Autodesk Inventor part; units mm, degrees
ref_plane "YZ Plane" through (0, 0, 0) normal (1, 0, 0) x (0, 1, 0)
ref_plane "XZ Plane" through (0, 0, 0) normal (0, 1, 0) x (-1, 0, 0)
ref_plane "XY Plane" through (0, 0, 0) normal (0, 0, 1) x (1, 0, 0)
sketch "草圖8" plane through (0, 0, 0) normal (0, 1, 0) x (-1, 0, 0)
  line L0 (10, 10) -> (-10, 10)
  line L1 (-10, 10) -> (-10, -10)
  line L2 (-10, -10) -> (10, -10)
  line L3 (10, -10) -> (10, 10)
  line L4 (10, 10) -> (-10, -10) construction
  line L5 (-10, 10) -> (10, -10) construction
  point P0 (0, 0)
  dimension "d36" = 20
  dimension "d37" = 20
extrude "擠出8" add sketch "草圖8" along normal blind 1.5
sketch "草圖9" plane through (0, 1.5, 0) normal (0, 1, 0) x (1, 0, 0)
  line L0 (-8, -7) -> (8, -7)
  line L1 (8, -7) -> (8, 7)
  line L2 (8, 7) -> (-8, 7)
  line L3 (-8, 7) -> (-8, -7)
  line L4 (-8, -7) -> (8, 7) construction
  line L5 (8, -7) -> (-8, 7) construction
  line L6 (-7, 6) -> (7, 6)
  line L7 (7, 6) -> (7, -6)
  line L8 (7, -6) -> (-7, -6)
  line L9 (-7, -6) -> (-7, 6)
  line L10 (-7, 6) -> (7, -6) construction
  line L11 (7, 6) -> (-7, -6) construction
  point P0 (0, 0)
  dimension "d40" = 16
  dimension "d41" = 14
  dimension "d46" = 14
  dimension "d47" = 12
extrude "擠出10" add sketch "草圖9" along normal blind 15
sketch "草圖11" plane through (-8, 1.5, 7) normal (0, 0, 1) x (1, 0, 0)
  line L0 (5.5, 18) -> (10.5, 18)
  line L1 (10.5, 18) -> (10.5, 12)
  line L2 (10.5, 12) -> (5.5, 12)
  line L3 (5.5, 12) -> (5.5, 18)
  line L4 (16, 15) -> (0, 15)
  line L5 (5.5, 18) -> (10.5, 12) construction
  line L6 (10.5, 18) -> (5.5, 12) construction
  point P0 (8, -1.5)
  point P1 (8, 15)
  point P2 (10.5, 15)
  point P3 (5.5, 15)
  dimension "d50" = 5
  dimension "d51" = 6
extrude "擠出11" cut sketch "草圖11" against normal blind 15 contours L4 L1 L2 L3
sketch "草圖12" plane through (0, 1.5, 0) normal (0, 1, 0) x (1, 0, 0)
  line L0 (-4.5, 2.5) -> (-2.5, 2.5)
  line L1 (-2.5, 2.5) -> (-2.5, -2.5)
  line L2 (-2.5, -2.5) -> (-4.5, -2.5)
  line L3 (-4.5, -2.5) -> (-4.5, 2.5)
  line L4 (-4.5, 2.5) -> (-2.5, -2.5) construction
  line L5 (-2.5, 2.5) -> (-4.5, -2.5) construction
  line L6 (2.5, 2.5) -> (4.5, 2.5)
  line L7 (4.5, 2.5) -> (4.5, -2.5)
  line L8 (4.5, -2.5) -> (2.5, -2.5)
  line L9 (2.5, -2.5) -> (2.5, 2.5)
  line L10 (2.5, 2.5) -> (4.5, -2.5) construction
  line L11 (4.5, 2.5) -> (2.5, -2.5) construction
  line L12 (7, 6) -> (7, -6)
  point P0 (0, 0)
  point P1 (-3.5, 0)
  point P2 (3.5, 0)
  point P3 (7, 0)
  dimension "d54" = 5
  dimension "d55" = 2
  dimension "d56" = 5
  dimension "d57" = 2
  dimension "d58" = 3.5
  dimension "d59" = 3.5
  dimension "d60" = 3.5
extrude "擠出12" add sketch "草圖12" along normal blind 1
properties part number "差分線圈激勵"
Design review of the part built by this model. Coordinates are the model's own, in mm. A direction names the side the tool comes from. Give positions to 0.01 mm unless a question says otherwise; leave off trailing zeros. Write each loop counter-clockwise with the first axis right and the second up, starting at its lowest first coordinate (ties: lowest second). Pieces come first, ordered by that corner, then holes. Notation, with made-up numbers: M -8.75,-10.75 L 47.25,-10.75 A19 cw 47.25,2.25 Z; hole C -22,-19 d3. An arc over 180 degrees is marked long. Return JSON: item names as keys, results as strings. Group by question number.
Item 1: Take a section at B-B (y = 14.5). Give the boundary of the cut face in (x, z).
Item 2: Tool access review of faces 4 (the flat face through (2.5, 15, -6.5)), 5 (the flat face through (-7, 9, 0)), 6 (the flat face through (0, 9, -7)): name each direction out of +Z, -Z, +X, -X, +Y, -Y from which nothing blocks a thin tool from reaching the whole face with its end or side.
Item 3: The part is to be moulded in two halves that separate along Z. For faces 1 (the flat face through (3, 2, -2.5)), 2 (the flat face through (2.5, 15, 6.5)), 3 (the flat face through (0, 9, 7)), say which applies: pulls with the +Z half, pulls with the -Z half, needs draft (parallel to the pull), parting line crosses it, or undercut.
Item 4: Take a section at A-A (y = 2). Give the boundary of the cut face in (x, z), plus the area to 3 significant figures.
Item 5: Clearance check with flat-ended pins moving along their axes: pin 1 Ø4.5 at (x, y) = (-0.5, 9.5) entering from +Z; pin 2 Ø5 at (x, y) = (-8, 11) entering from -Z; pin 3 Ø3 at (y, z) = (10.5, 3.5) entering from +X. State where each tip first meets the part, or that it passes through.
Item 6: Wall thickness on line 1 along Z through (x, y) = (2, 7.25); line 2 along X through (y, z) = (10.25, -1); line 3 along Y through (x, z) = (8, -7.5): over which ranges is each line inside the solid? List them lowest first.
Item 7: Take a section at D-D (z = 6.5). Give the boundary of the cut face in (x, y), plus the area to 3 significant figures.
Item 8: Take a section at C-C (x = 3). Give the boundary of the cut face in (y, z), plus the area to 3 significant figures.
Return value:
{
 "1": {"outline": "M -8,-7 L -2.5,-7 L -2.5,-6 L -7,-6 L -7,6 L -2.5,6 L -2.5,7 L -8,7 Z; M 2.5,-7 L 8,-7 L 8,7 L 2.5,7 L 2.5,6 L 7,6 L 7,-6 L 2.5,-6 Z"},
 "2": {"face 4": "+Z, -Z, +Y", "face 5": "+Y", "face 6": "-Z, +X, -X, +Y"},
 "3": {"face 1": "undercut", "face 2": "needs draft", "face 3": "pulls with the +Z half"},
 "4": {"outline": "M -8,-7 L 8,-7 L 8,7 L -8,7 Z; M -4.5,-2.5 L -2.5,-2.5 L -2.5,2.5 L -4.5,2.5 Z; M 2.5,-2.5 L 4.5,-2.5 L 4.5,2.5 L 2.5,2.5 Z; hole M -7,-6 L 7,-6 L 7,6 L -7,6 Z", "area": "76.0 mm2"},
 "5": {"pin 1": "stops at z = 7", "pin 2": "stops at z = -7", "pin 3": "stops at x = 8"},
 "6": {"line 1": "z = -7 to -6, 6 to 7", "line 2": "x = -8 to -7, 7 to 8", "line 3": "y = 0 to 1.5"},
 "7": {"outline": "M -10,0 L 10,0 L 10,1.5 L 8,1.5 L 8,16.5 L 2.5,16.5 L 2.5,13.5 L -2.5,13.5 L -2.5,16.5 L -8,16.5 L -8,1.5 L -10,1.5 Z", "area": "255 mm2"},
 "8": {"outline": "M 0,-10 L 1.5,-10 L 1.5,-7 L 16.5,-7 L 16.5,-6 L 1.5,-6 L 1.5,-2.5 L 2.5,-2.5 L 2.5,2.5 L 1.5,2.5 L 1.5,6 L 16.5,6 L 16.5,7 L 1.5,7 L 1.5,10 L 0,10 Z", "area": "65.0 mm2"}
}
